from build123d import *

# Parameters (mm, degrees)
F0_R         = 25
F1_DEPTH     = 10
F2_W         = 0.9488426149
F2_H         = 1.2651239522
F2_W_2       = 6.0093384236
F2_H_2       = 3.584517166
F2_W_3       = 3.9007980376
F2_H_3       = 1.8976870924
F2_W_4       = 4.6387878247
F2_H_4       = 4.0062256157
F2_W_5       = 1.7922576517
F2_H_5       = 3.0573830009
F2_W_6       = 7.0636067539
F2_H_6       = 7.4619053196
F2_W_7       = 3.1628105789
F2_H_7       = 4.8496406525
F2_W_8       = 2.3193918169
F2_H_8       = 10.2264162851
F2_W_9       = 9.2775728554
F2_H_9       = 7.0636067539
F2_W_10      = 22.1396633424
F2_H_10      = 4.6387854964
F2_W_11      = 2.7022243196
F2_H_11      = 4.5333597809
F2_W_12      = 0.7379893214
F2_H_12      = 1.8976833671
F2_W_13      = 4.3890562559
F2_H_13      = 8.9737139642
F2_W_14      = 1.7922595143
F2_H_14      = 1.7922581173
F3_DEPTH     = 3
F4_T1_DEPTH  = 60
F4_T6_DEPTH  = 60
F4_T12_DEPTH = 60
F4_T18_DEPTH = 60


# Not quite as in the source:
# - a fillet or chamfer that OpenCascade refuses, or shapes differently, is made with other operations: its cross-section is extruded or revolved along the edge and cut away or added


with BuildPart() as f1:
    # F0 (on Front) → F1 (new body)
    with BuildSketch(Plane.XZ):
        Polygon((-25.3573476618, 34.1470630352), (-40.3116381718, -13.5642479438), (0.4433851295, -42.5302292964), (40.5856652519, -12.7208793106), (24.6399354522, 34.6682935156), align=None)
        Circle(F0_R, mode=Mode.SUBTRACT)
    extrude(amount=F1_DEPTH)

    # F2 (on face) → F3 (join)
    with BuildSketch(Plane.XZ.offset(10)):
        with Locations((-30.2208252251, -4.310084274)):
            Rectangle(F2_W, F2_H)
        with Locations((-29.0611283854, -11.6899730638)):
            Rectangle(F2_W_2, F2_H_2)
        with Locations((-18.5184301808, -23.0760863051)):
            Rectangle(F2_W_3, F2_H_3)
        with Locations((0.6165653467, -30.455974862)):
            Rectangle(F2_W_4, F2_H_4)
        with Locations((16.7996054515, -25.0264853239)):
            Rectangle(F2_W_5, F2_H_5)
        with Locations((33.0353630707, -9.833295284)):
            Rectangle(F2_W_6, F2_H_6)
        with Locations((23.7050717697, -18.6481522396)):
            Rectangle(F2_W_7, F2_H_7)
        with Locations((27.3950155824, 7.0233154693)):
            Rectangle(F2_W_8, F2_H_8)
        with Locations((18.2228693739, 27.1598668769)):
            Rectangle(F2_W_9, F2_H_9)
        with Locations((-11.9292445015, 29.2156925425)):
            Rectangle(F2_W_10, F2_H_10)
        with Locations((-26.7084598216, 16.9334514067)):
            Rectangle(F2_W_11, F2_H_11)
        with Locations((-18.5184301808, 21.3086707518)):
            Rectangle(F2_W_12, F2_H_12)
        with Locations((-27.5518757897, 4.4868569821)):
            Rectangle(F2_W_13, F2_H_13)
        with Locations((-35.9138809144, -8.3690227475)):
            Rectangle(F2_W_14, F2_H_14)
    extrude(amount=F3_DEPTH)

    # F4: fillet of radius 2 on 2 edges, made by hand

    # F4_s2 → F4_t1 (cut)
    with BuildSketch(Plane(origin=(-24.4530139807, 0, 17.3795888115), x_dir=(0, 1, 0), z_dir=(0.815100466, 0, -0.5793196271))):
        with BuildLine():
            ThreePointArc((-8, -34.4095480118), (-9.4142135624, -33.8237615742), (-10, -32.4095480118))
            Line((-10, -32.4095480118), (-10, -34.4095480118))
            Line((-10, -34.4095480118), (-8, -34.4095480118))
        make_face()
    extrude(amount=F4_T1_DEPTH, mode=Mode.SUBTRACT)


with BuildPart() as f4_tool4:
    # F4_s5 → F4_t6 (new body)
    with BuildSketch(Plane(origin=(-24.0853680735, 0, -17.8856099914), x_dir=(0, 1, 0), z_dir=(0.8028456024, 0, 0.5961869997))):
        with BuildLine():
            ThreePointArc((-10, -32.4095480118), (-9.4142135624, -33.8237615742), (-8, -34.4095480118))
            Line((-8, -34.4095480118), (-10, -34.4095480118))
            Line((-10, -34.4095480118), (-10, -32.4095480118))
        make_face()
    extrude(amount=F4_T6_DEPTH)

    split(bisect_by=Plane.XY.offset(-13.5642479438), keep=Keep.BOTTOM)

    split(bisect_by=Plane.YZ.offset(36.5671664476), keep=Keep.BOTTOM)


with BuildPart() as f1_1:
    add(f1.part)

    # F4_t3: cut F4_tool4
    add(f4_tool4.part, mode=Mode.SUBTRACT)


with BuildPart() as f4_tool10:
    # F4_s11 → F4_t12 (new body)
    with BuildSketch(Plane(origin=(-24.0853680735, 0, -17.8856099914), x_dir=(0, 1, 0), z_dir=(0.8028456024, 0, 0.5961869997))):
        with BuildLine():
            ThreePointArc((-10, -32.4095480118), (-9.4142135624, -33.8237615742), (-8, -34.4095480118))
            Line((-8, -34.4095480118), (-10, -34.4095480118))
            Line((-10, -34.4095480118), (-10, -32.4095480118))
        make_face()
    extrude(amount=F4_T12_DEPTH)

    split(bisect_by=Plane.XY.offset(-13.5642479438), keep=Keep.BOTTOM)

    split(bisect_by=Plane.YZ.offset(36.5671664476), keep=Keep.TOP)


with BuildPart() as f1_2:
    add(f1_1.part)

    # F4_t9: cut F4_tool10
    add(f4_tool10.part, mode=Mode.SUBTRACT)


with BuildPart() as f4_tool16:
    # F4_s17 → F4_t18 (new body)
    with BuildSketch(Plane(origin=(-24.0853680735, 0, -17.8856099914), x_dir=(0, 1, 0), z_dir=(0.8028456024, 0, 0.5961869997))):
        with BuildLine():
            ThreePointArc((-10, -32.4095480118), (-9.4142135624, -33.8237615742), (-8, -34.4095480118))
            Line((-8, -34.4095480118), (-10, -34.4095480118))
            Line((-10, -34.4095480118), (-10, -32.4095480118))
        make_face()
    extrude(amount=F4_T18_DEPTH)

    split(bisect_by=Plane.XY.offset(-13.5642479438), keep=Keep.TOP)

    split(bisect_by=Plane.YZ.offset(36.5671664476), keep=Keep.TOP)


with BuildPart() as f1_3:
    add(f1_2.part)

    # F4_t15: cut F4_tool16
    add(f4_tool16.part, mode=Mode.SUBTRACT)


solid = f1_3.part
The model under review builds one solid part; all positions refer to its coordinate system, in mm. A direction names the side the tool comes from. Round coordinates to 2 decimals unless told otherwise and drop trailing zeros. Loops run counter-clockwise (first coordinate to the right, second up) from the corner with the lowest first, then second, coordinate; pieces in that order, holes last. Notation, with made-up numbers: (21.25, 11) -> (59.25, 11) arc R28 cw to (59.25, 37) -> close; hole circle Ø3 at (78, 7.25). An arc over 180 degrees is marked (long way). Return JSON: item names as keys, results as strings.
(1) Add section C-C on y = -9. Write out the cut boundary in (x, z), plus the area to 3 significant figures.
Solved:
{"outline": "(-40.23, -13.3) -> (0.44, -42.2) -> (40.5, -12.45) -> (24.64, 34.67) -> (-25.36, 34.15) -> close; hole circle Ø50 at (0, 0)", "area": "2,310 mm2"}
(2) Add section A-A on y = -2. Write out the cut boundary in (x, z), plus the area to 3 significant figures.
Solved:
{"outline": "(-40.31, -13.56) -> (0.44, -42.53) -> (40.59, -12.72) -> (24.64, 34.67) -> (-25.36, 34.15) -> close; hole circle Ø50 at (0, 0)", "area": "2,340 mm2"}
(3) For faces 4 (the flat face through (-28.06, -11, 17)), 5 (the flat face through (-22.999, -11, 29)), 6 (the flat face through (-28, -11, 8.974)), 7 (the flat face through (18, -11, 30.692)), 8 (the flat face through (13.584, -11, 27)), list the 3-axis set-ups (+Z, -Z, +X, -X, +Y, -Y) from which the entire face can be reached by the end or side of a thin tool; tool diameter is ignored.
Solved:
{"face 4": "+Z, -X, -Y", "face 5": "+Z, -Z, -X, -Y", "face 6": "-X, -Y", "face 7": "+Z, +X, -Y", "face 8": "+Z, -Z, -Y"}
(4) Add section B-B on z = 10. Write out the cut boundary in (x, y).
Solved:
{"outline": "(-32.93, -10) -> (-22.91, -10) -> (-22.91, 0) -> (-32.93, 0) -> close; (22.91, -10) -> (26.24, -10) -> (26.24, -13) -> (28.55, -13) -> (28.55, -10) -> (32.94, -10) -> (32.94, 0) -> (22.91, 0) -> close"}
(5) For line 1 (Z direction, x = -27.5, y = -12); line 2 (Z direction, x = 0, y = -3); line 3 (X direction, y = -0.75, z = -17), list the stretches that pass through material, from the lowest coordinate up.
Solved:
{"line 1": "-13.48 to -9.9, 0 to 8.97, 14.67 to 19.2", "line 2": "-42.22 to -25, 25 to 34.41", "line 3": "-35.48 to -18.33, 18.33 to 34.82"}
(6) The part is to be moulded in two halves that separate along Z. For faces 1 (the flat face through (24, -11, -16.223)), 2 (the flat face through (-27, -13, 17)), 3 (the flat face through (-20, -4, -28)), say which applies: released by +Z, released by -Z, zero draft, split by the parting line, or undercut.
Solved:
{"face 1": "undercut", "face 2": "zero draft", "face 3": "released by -Z"}
(7) For pin 1 (3 mm diameter, centred on y = -8.5, z = 25, fed in from -X); pin 2 (3 mm diameter, centred on y = -2, z = 17.5, fed in from +X); pin 3 (2 mm diameter, centred on x = -30, z = -2, fed in from +Y); pin 4 (1.4 mm diameter, centred on x = -36, y = -12, fed in from -Z), all flat-tipped, find the tip position at first contact; note any pin that passes through.
Solved:
{"pin 1": "x = -28.69", "pin 2": "x = 30.92", "pin 3": "y = 0", "pin 4": "z = -9.27"}
